```python
from build123d import *

# Parameters (mm, degrees)
SKETCH1_W           = 685.8
SKETCH1_H           = 381
SKETCH1_W_2         = 615.95
SKETCH1_H_2         = 311.15
BOSS_EXTRUDE1_DEPTH = 12.7
FILLET1_R           = 3.175


with BuildPart() as part:
    # Sketch1 → Boss-Extrude1 (new body)
    with BuildSketch(Plane.ZY.offset(311.15)):
        with Locations((0, 330.2)):
            Rectangle(SKETCH1_W, SKETCH1_H)
        with Locations((0, 330.2)):
            Rectangle(SKETCH1_W_2, SKETCH1_H_2, mode=Mode.SUBTRACT)
    extrude(amount=BOSS_EXTRUDE1_DEPTH)

    # Fillet1
    fillet1_edges = [part.edges().sort_by_distance(p)[0] for p in [
        (-317.5, 485.775, -307.975),
        (-317.5, 174.625, -307.975),
        (-317.5, 174.625, 307.975),
        (-317.5, 485.775, 307.975),
        (-317.5, 520.7, -342.9),
        (-317.5, 520.7, 342.9),
        (-317.5, 139.7, 342.9),
        (-317.5, 139.7, -342.9),
    ]]
    fillet(fillet1_edges, radius=FILLET1_R)


solid = part.part
```
Design review of the part built by this model. Coordinates are the model's own, in mm. A direction names the side the tool comes from. Give positions to 0.01 mm unless a question says otherwise; leave off trailing zeros. Order: outer loops, then holes, each group sorted by start corner. A loop starts at its lowest first (then second) coordinate and runs counter-clockwise, first axis right, second up. Notation, with made-up numbers: (7, 67) -> (60, 67) arc R14 cw to (60, 87) -> close; hole circle Ø1 at (37, -11.75). An arc over 180 degrees is marked (long way). Write each question's results on one line, items separated by ' | '. Start each with the question number.
Q1. Mouldability with a two-part tool opening along Z and no side actions: class faces 3 (the flat face through (-317, 328, -342.9)), 4 (the flat face through (-317, 174.625, -4)), 5 (the flat face through (-317, 328, -307.975)), 6 (the flat face through (-317, 139.7, -5)) as +Z half, -Z half, draft (parallel to the pull), parting line (faces both ways), or undercut.
Q2. Add section A-A on y = 263.5. Give the boundary of the cut face in (x, z) (3 decimals).
Q3. Add section B-B on z = -285.5. Give the boundary of the cut face in (x, y) (3 decimals), and give its area (3 significant figures).
Q4. Machinability: for faces 1 (the flat face through (-317, 485.775, -4)), 2 (the flat face through (-317, 328, 342.9)), which of the approach directions +Z, -Z, +X, -X, +Y, -Y give a long, thin tool a straight path to every point of the face, cutting with its end or side? Answer none if there is none.
Q5. Wall thickness on L1, parallel to Z at x = -314.5, y = 231.5 (3 decimals); L2, parallel to Y at x = -318, z = 37 (3 decimals): over which ranges is each line inside the solid? List them lowest first. Write a range as from..to.
Q6. Add section C-C on x = -319. Give the boundary of the cut face in (y, z) (3 decimals).
Found:
1) face 3: -Z half | face 4: undercut | face 5: undercut | face 6: draft
2) outline: (-323.85, -342.9) -> (-311.15, -342.9) -> (-311.15, -307.975) -> (-323.85, -307.975) -> close; (-323.85, 307.975) -> (-311.15, 307.975) -> (-311.15, 342.9) -> (-323.85, 342.9) -> close
3) outline: (-323.85, 139.7) -> (-311.15, 139.7) -> (-311.15, 174.625) -> (-323.85, 174.625) -> close; (-323.85, 485.775) -> (-311.15, 485.775) -> (-311.15, 520.7) -> (-323.85, 520.7) -> close | area: 887 mm2
4) face 1: +X, -X | face 2: +Z, +X, -X, +Y, -Y
5) L1: z = -342.9..-307.975, 307.975..342.9 | L2: y = 139.7..174.625, 485.775..520.7
6) outline: (139.7, -339.725) arc R3.175 ccw to (142.875, -342.9) -> (517.525, -342.9) arc R3.175 ccw to (520.7, -339.725) -> (520.7, 339.725) arc R3.175 ccw to (517.525, 342.9) -> (142.875, 342.9) arc R3.175 ccw to (139.7, 339.725) -> close; hole (174.625, -304.8) arc R3.175 ccw to (177.8, -307.975) -> (482.6, -307.975) arc R3.175 ccw to (485.775, -304.8) -> (485.775, 304.8) arc R3.175 ccw to (482.6, 307.975) -> (177.8, 307.975) arc R3.175 ccw to (174.625, 304.8) -> close
